Part model, mm, in its own coordinate system. A direction names the side the tool comes from. Give positions to 0.01 mm unless a question says otherwise; leave off trailing zeros. Order: outer loops, then holes, each group sorted by start corner. A loop starts at its lowest first (then second) coordinate and runs counter-clockwise, first axis right, second up. Notation, with made-up numbers: M -3,-23 L 4,-23 A20 cw 4,5 Z; hole C 38,84 d7. An arc over 180 degrees is marked long. Return JSON: item names as keys, results as strings.
from build123d import *

# Parameters (mm, degrees)
F0_W      = 55.85
F0_H      = 3
F1_DEPTH  = 87.49
F2_T      = -0.75
F3_DEPTH  = 0.75
F4_W      = 20
F4_H      = 7
F4_W_2    = 16
F4_H_2    = 3
F5_DEPTH  = 0.75
F7_ANGLE  = 90
F8_ANGLE  = 90
F10_ANGLE = 90
F11_ANGLE = 90
F12_R     = 1.5
F13_R     = 1.5
F15_ANGLE = 90
F16_DEPTH = 1
F17_R     = 1.5
F18_R     = 1.5
F19_R     = 1.49999
F20_R     = 1.49999
F21_R     = 4
F22_R     = 4
F23_W     = 55.85
F23_H     = 87.49
F24_DEPTH = 4
F25_T     = -0.25
F26_R     = 9.693411876
F27_DEPTH = 0.25
F29_R     = 1.375
F30_DEPTH = 1.74


# Not quite as in the source:
# - a fillet or chamfer is up to 0.001 mm smaller than in the source, because OpenCascade refuses the exact size


with BuildPart() as f1:
    # F0 (on Front) → F1 (new body)
    with BuildSketch(Plane.XZ):
        with Locations((-39.0305130277, -21.5327367023)):
            Rectangle(F0_W, F0_H)
    extrude(amount=-F1_DEPTH)

    # F2
    f2_openings = [f1.faces().sort_by_distance(p)[0] for p in [
        (-39.030513, 43.745, -20.032737),
    ]]
    offset(amount=F2_T, openings=f2_openings)

    # F3 (cut): a face of the model
    f3_faces = [f1.faces().sort_by_distance(p)[0] for p in [
        (-39.0305130277, 86.74, -21.1577367023),
    ]]
    extrude(f3_faces, amount=-F3_DEPTH, mode=Mode.SUBTRACT)

    # F4 (on face) → F5 (join, through all)
    with BuildSketch(Plane.XY.offset(-22.2827367023)):
        with Locations((-39.0305130277, 90.99)):
            Rectangle(F4_W, F4_H)
        with Locations((-39.0305130277, 90.99)):
            Rectangle(F4_W_2, F4_H_2, mode=Mode.SUBTRACT)
    extrude(amount=-F5_DEPTH)

    # F6 (on face) → F7 (revolve)
    with BuildSketch(Plane.YZ.offset(-66.2055130277)):
        with BuildLine():
            Line((82.49, -21.0327367023), (83.365, -21.0327367023))
            ThreePointArc((83.365, -21.0327367023), (82.49, -20.1577367023), (81.615, -21.0327367023))
            Line((81.615, -21.0327367023), (82.49, -21.0327367023))
        make_face()
    revolve(axis=Axis((-66.2055130277, 82.0525, -21.0327367023), (0, 1, 0)), revolution_arc=F7_ANGLE)

    # F6 (on face) → F8 (revolve)
    with BuildSketch(Plane.YZ.offset(-66.2055130277)):
        with BuildLine():
            Line((27.49, -21.0327367023), (28.365, -21.0327367023))
            ThreePointArc((28.365, -21.0327367023), (27.49, -20.1577367023), (26.615, -21.0327367023))
            Line((26.615, -21.0327367023), (27.49, -21.0327367023))
        make_face()
    revolve(axis=Axis((-66.2055130277, 27.0525, -21.0327367023), (0, 1, 0)), revolution_arc=F8_ANGLE)

    # F9 (on face) → F10 (revolve)
    with BuildSketch(Plane(origin=(-11.8555130277, 0, 0), x_dir=(0, -1, 0), z_dir=(-1, 0, 0))):
        with BuildLine():
            Line((-83.365, -21.0327367023), (-81.615, -21.0327367023))
            ThreePointArc((-81.615, -21.0327367023), (-82.49, -20.1577367023), (-83.365, -21.0327367023))
        make_face()
    revolve(axis=Axis((-11.8555130277, 82.49, -21.0327367023), (0, -1, 0)), revolution_arc=F10_ANGLE)

    # F9 (on face) → F11 (revolve)
    with BuildSketch(Plane(origin=(-11.8555130277, 0, 0), x_dir=(0, -1, 0), z_dir=(-1, 0, 0))):
        with BuildLine():
            Line((-28.365, -21.0327367023), (-26.615, -21.0327367023))
            ThreePointArc((-26.615, -21.0327367023), (-27.49, -20.1577367023), (-28.365, -21.0327367023))
        make_face()
    revolve(axis=Axis((-11.8555130277, 27.49, -21.0327367023), (0, -1, 0)), revolution_arc=F11_ANGLE)

    # F12
    f12_edges = [f1.edges().sort_by_distance(p)[0] for p in [
        (-66.205513, 0.75, -21.157737),
    ]]
    fillet(f12_edges, radius=F12_R)

    # F13
    f13_edges = [f1.edges().sort_by_distance(p)[0] for p in [
        (-11.855513, 0.75, -21.157737),
    ]]
    fillet(f13_edges, radius=F13_R)

    # F14 (on face) → F15 (revolve)
    with BuildSketch(Plane(origin=(0, 0.75, 0), x_dir=(-1, 0, 0), z_dir=(0, 1, 0))):
        with BuildLine():
            Line((38.1555130277, -21.0327367023), (39.9055130277, -21.0327367023))
            ThreePointArc((39.9055130277, -21.0327367023), (39.0305130277, -20.1577367023), (38.1555130277, -21.0327367023))
        make_face()
    revolve(axis=Axis((-39.0305130277, 0.75, -21.0327367023), (-1, 0, 0)), revolution_arc=F15_ANGLE)

    # F16 (add): a face of the model
    f16_faces = [f1.faces().sort_by_distance(p)[0] for p in [
        (-39.0305130277, 44.6180943483, -23.0327367023),
    ]]
    extrude(f16_faces, amount=F16_DEPTH)

    # F17
    f17_edges = [f1.edges().sort_by_distance(p)[0] for p in [
        (-47.030513, 89.49, -23.157737),
    ]]
    fillet(f17_edges, radius=F17_R)

    # F18
    f18_edges = [f1.edges().sort_by_distance(p)[0] for p in [
        (-31.030513, 89.49, -23.157737),
    ]]
    fillet(f18_edges, radius=F18_R)

    # F19 (radius 1.5 in the source; OpenCascade refuses exactly that, so slightly less here)
    f19_edges = [f1.edges().sort_by_distance(p)[0] for p in [
        (-31.030513, 92.49, -23.157737),
    ]]
    fillet(f19_edges, radius=F19_R)

    # F20 (radius 1.5 in the source; OpenCascade refuses exactly that, so slightly less here)
    f20_edges = [f1.edges().sort_by_distance(p)[0] for p in [
        (-47.030513, 92.49, -23.157737),
    ]]
    fillet(f20_edges, radius=F20_R)

    # F21
    f21_edges = [f1.edges().sort_by_distance(p)[0] for p in [
        (-29.030513, 94.49, -23.157737),
    ]]
    fillet(f21_edges, radius=F21_R)

    # F22
    f22_edges = [f1.edges().sort_by_distance(p)[0] for p in [
        (-49.030513, 94.49, -23.157737),
    ]]
    fillet(f22_edges, radius=F22_R)


with BuildPart() as f24:
    # F23 (on face) → F24 (new body)
    with BuildSketch(Plane(origin=(0, 0, -24.0327367023), x_dir=(1, 0, 0), z_dir=(0, 0, -1))):
        with Locations((-39.0305130277, -43.745)):
            Rectangle(F23_W, F23_H)
    extrude(amount=F24_DEPTH)

    # F25
    f25_openings = [f24.faces().sort_by_distance(p)[0] for p in [
        (-39.030513, 87.49, -26.032737),
    ]]
    offset(amount=F25_T, openings=f25_openings)

    # F26 (on face) → F27 (cut, through all)
    with BuildSketch(Plane(origin=(0, 0, -28.0327367023), x_dir=(1, 0, 0), z_dir=(0, 0, -1))):
        with Locations((-39.0305130277, -43.745)):
            Circle(F26_R)
    extrude(amount=-F27_DEPTH, mode=Mode.SUBTRACT)

    # F29 (on face) → F30 (join)
    with BuildSketch(Plane.XY.offset(-24.0327367023)):
        with Locations((-51.9555130277, 15)):
            Circle(F29_R)
        with Locations((-26.1055130277, 15)):
            Circle(F29_R)
        with Locations((-26.1055130277, 72.49)):
            Circle(F29_R)
        with Locations((-51.9555130277, 72.49)):
            Circle(F29_R)
    extrude(amount=F30_DEPTH)


solid = f24.part
Q1. 3-axis set-ups, long thin cutter, end or side, ignore diameter. For faces 1 (the flat face through (-11.106, 44, -26)), 2 (the cylindrical face through (-27.48, 72.55, -23.17)), 3 (the flat face through (-39.4, 33.6, -27.783)): which of +Z, -Z, +X, -X, +Y, -Y reach the whole face in a straight line?
Established:
{"face 1": "+Z, -Z, +X, +Y, -Y", "face 2": "+Z", "face 3": "+Y"}
Q2. Pin check, flat tips, straight feed: pin 1 (1 mm diameter, centred on x = -40, z = -27, fed in from +Y); pin 2 (11.5 mm diameter, centred on x = -39.03, y = 43.74, fed in from -Z); pin 3 (1.5 mm diameter, centred on x = -36, z = -23, fed in from +Y). Stop position of each tip, or through.
Established:
{"pin 1": "stops at y = 0.25", "pin 2": "stops at z = -24.28", "pin 3": "passes through"}
Q3. Band-saw the part on A-A (y = 6). Give the cut face in (x, z), then the cut area to 3 significant figures.
Established:
{"outline": "M -66.96,-28.03 L -11.11,-28.03 L -11.11,-24.03 L -66.96,-24.03 Z; hole M -66.71,-27.78 L -11.36,-27.78 L -11.36,-24.28 L -66.71,-24.28 Z", "area": "29.7 mm²"}
Q4. Two-plate mould, pull along Y, no slides. Class faces 4 (the flat face through (-66.706, 44, -26)), 5 (the flat face through (-39, 0.25, -26)), 6 (the cylindrical face through (-27.48, 15.06, -23.17)): +Y half, -Y half, draft (parallel to the pull), parting line (faces both ways), or undercut.
Established:
{"face 4": "draft", "face 5": "+Y half", "face 6": "undercut"}
Q5. Probe line 1 along Z through (x, y) = (-31.5, 60); line 2 along X through (y, z) = (73, -27.3); line 3 along Y through (x, z) = (-13.5, -27.45). List the from-to ranges inside material, lowest first.
Established:
{"line 1": "z = -28.03 to -27.78, -24.28 to -24.03", "line 2": "x = -66.96 to -66.71, -11.36 to -11.11", "line 3": "y = 0 to 0.25"}
Q6. Band-saw the part on D-D (x = -43.5). Give the cut face in (y, z), then the cut area to 3 significant figures.
Established:
{"outline": "M 0,-28.03 L 35.14,-28.03 L 35.14,-27.78 L 0.25,-27.78 L 0.25,-24.28 L 87.49,-24.28 L 87.49,-24.03 L 0,-24.03 Z; M 52.35,-28.03 L 87.49,-28.03 L 87.49,-27.78 L 52.35,-27.78 Z", "area": "40.3 mm²"}
Q7. Band-saw the part on C-C (z = -26.3). Give the cut face in (x, y).
Established:
{"outline": "M -66.96,0 L -11.11,0 L -11.11,87.49 L -11.36,87.49 L -11.36,0.25 L -66.71,0.25 L -66.71,87.49 L -66.96,87.49 Z"}
Q8. Band-saw the part on B-B (x = -55). Give the cut face in (y, z).
Established:
{"outline": "M 0,-28.03 L 87.49,-28.03 L 87.49,-27.78 L 0.25,-27.78 L 0.25,-24.28 L 87.49,-24.28 L 87.49,-24.03 L 0,-24.03 Z"}
